Autodesk Inventor part; units mm, degrees
ref_plane "YZ Plane" through (0, 0, 0) normal (1, 0, 0) x (0, 1, 0)
ref_plane "XZ Plane" through (0, 0, 0) normal (0, 1, 0) x (-1, 0, 0)
ref_plane "XY Plane" through (0, 0, 0) normal (0, 0, 1) x (1, 0, 0)
sketch "スケッチ1" plane through (0, 0, 0) normal (0, 0, 1) x (1, 0, 0)
  line L0 (-21.75, 5.5) -> (-21.75, -5.5)
  line L1 (-21.75, -5.5) -> (-19.75, -5.5)
  line L2 (-21.75, 5.5) -> (-19.75, 5.5)
  line L3 (-19.75, 7.6) -> (-19.75, 10.5)
  line L4 (-19.75, 10.5) -> (19.75, 10.5)
  line L5 (19.75, 10.5) -> (19.75, 7.6)
  line L6 (-19.75, -7.6) -> (-19.75, -10.5)
  line L7 (-19.75, -10.5) -> (19.75, -10.5)
  line L8 (19.75, -10.5) -> (19.75, -7.6)
  line L9 (19.75, 5.5) -> (21.75, 5.5)
  line L10 (21.75, 5.5) -> (21.75, -5.5)
  line L11 (21.75, -5.5) -> (19.75, -5.5)
  line L12 (0, 0) -> (0, 10.5) construction
  line L13 (0, 0) -> (-21.75, 0) construction
  arc A0 (-19.75, 5.5) -> (-19.75, 7.6) centre (-19.75, 6.55) ccw
  arc A1 (-19.75, -7.6) -> (-19.75, -5.5) centre (-19.75, -6.55) ccw
  arc A2 (19.75, 7.6) -> (19.75, 5.5) centre (19.75, 6.55) ccw
  arc A3 (19.75, -5.5) -> (19.75, -7.6) centre (19.75, -6.55) ccw
  circle A4 centre (0, 0) radius 2.25
  dimension "d0" = 39.5
  dimension "d1" = 2
  dimension "d2" = 11
  dimension "d8" = 1.05
  dimension "d10" = 5
  dimension "d12" = 4.5
extrude "押し出し1" add sketch "スケッチ1" along normal blind 3
sketch "スケッチ2" plane through (0, 0, 0) normal (0, 0, -1) x (-1, 0, 0)
  circle A0 centre (0, 0) radius 2.25
  line L0 (-19.75, 10.5) -> (19.75, 10.5)
  line L1 (-21.75, -5.5) -> (-21.75, 5.5)
  arc A1 (6.3246, 3) -> (-6.3246, 3) centre (0, 0) ccw
  line L2 (-6.3246, 3) -> (-11.75, 3)
  line L3 (-11.75, 3) -> (-23.9536, 14.4408)
  line L4 (-23.9536, 14.4408) -> (23.9536, 14.4408)
  line L5 (23.9536, 14.4408) -> (11.75, 3)
  line L6 (11.75, 3) -> (6.3246, 3)
  line L7 (-19.75, 10.5) -> (19.75, 10.5) construction
  line L8 (0, 10.5) -> (0, 0) construction
  line L9 (0, 0) -> (-21.75, 0) construction
  arc A2 (-6.3246, -3) -> (6.3246, -3) centre (0, 0) ccw
  line L10 (-6.3246, -3) -> (-11.75, -3)
  line L11 (-11.75, -3) -> (-23.9536, -14.4408)
  line L12 (-23.9536, -14.4408) -> (23.9536, -14.4408)
  line L13 (23.9536, -14.4408) -> (11.75, -3)
  line L14 (11.75, -3) -> (6.3246, -3)
  dimension "d17" = 7
  dimension "d19" = 3
  dimension "d38" = 8
extrude "押し出し2" cut sketch "スケッチ2" against normal blind 10 contours L3 L4 L5 L0 | L0 L5 L6 A1 L2 L3 | A2 L14 L13 L12 L11 L10
fillet "フィレット1" radius 2 8 edges at (6.3246, 3, 1.5) (-6.3246, 3, 1.5) (6.3246, -3, 1.5) (-6.3246, -3, 1.5) (11.75, -3, 1.5) (11.75, 3, 1.5) (-11.75, 3, 1.5) (-11.75, -3, 1.5)
sketch "スケッチ3" plane through (0, 0, 3) normal (0, 0, 1) x (1, 0, 0)
  circle A0 centre (0, 0) radius 2.25
  line L0 (2.75, 1.5877) -> (2.75, -1.5877)
  line L1 (2.75, -1.5877) -> (0, -3.1754)
  line L2 (0, -3.1754) -> (-2.75, -1.5877)
  line L3 (-2.75, -1.5877) -> (-2.75, 1.5877)
  line L4 (-2.75, 1.5877) -> (0, 3.1754)
  line L5 (0, 3.1754) -> (2.75, 1.5877)
  line L6 (0, 3.187) -> (-2.76, 1.5935)
  line L7 (-2.76, 1.5935) -> (-2.76, -1.5935)
  line L8 (-2.76, -1.5935) -> (0, -3.187)
  line L9 (0, -3.187) -> (2.76, -1.5935)
  line L10 (2.76, -1.5935) -> (2.76, 1.5935)
  line L11 (2.76, 1.5935) -> (0, 3.187)
  circle A1 centre (0, 2.137) radius 1.05
  circle A2 centre (-1.8507, 1.0685) radius 1.05
  circle A3 centre (-1.8507, -1.0685) radius 1.05
  circle A4 centre (0, -2.137) radius 1.05
  circle A5 centre (1.8507, -1.0685) radius 1.05
  circle A6 centre (1.8507, 1.0685) radius 1.05
  point P0 (-2.76, 1.5935)
  point P1 (-2.76, -1.5935)
  point P2 (0, -3.187)
  point P3 (2.76, -1.5935)
  point P4 (2.76, 1.5935)
  dimension "d47" = 2.1
  dimension "d46" = 5.5
  dimension "d48" = 0.01
  dimension "d51" = 360
extrude "押し出し3" cut sketch "スケッチ3" against normal blind 2.2
equation "\"d2\" = d3"
equation "\"d10\" = d27"
properties part number "足首_サブフレーム_1_3" material "アルミニウム 2014-T4"
Here's how the part is built. I have some questions about the finished solid (model axes, mm). A direction names the side the tool comes from. Coordinates: 2 decimals unless noted, no trailing zeros. Write each loop counter-clockwise with the first axis right and the second up, starting at its lowest first coordinate (ties: lowest second). Pieces come first, ordered by that corner, then holes.
Item 1: I want a section at D-D on y = 8. Write out the boundary of the cut face in (x, z).
Item 2: If I drill on line 1 (X direction, y = 0, z = 0.25); line 2 (X direction, y = 1, z = 2.65); line 3 (Y direction, x = -9.5, z = 0.85), over which ranges is the centre line in solid material (lowest first)?
Item 3: On a 3-axis mill with a long thin cutter (end or side, diameter ignored), from which of +Z, -Z, +X, -X, +Y, -Y can I reach the whole of each face in a straight line? I mean faces 1 (the cylindrical face through (-6.53, -3.24, 1.52)), 2 (the flat face through (-16.09, 7.07, 1.48)), 3 (the flat face through (21, 5.5, 1)), 4 (the flat face through (-21, 5.5, 1)), 5 (the flat face through (-21, -5.5, 1)). Say none if no direction works.
Item 4: Will these pins go through, and if not, where does the flat tip stop? pin 1 (0.9 mm diameter, centred on x = -8.5, z = 1.5, fed in from -Y); pin 2 (12 mm diameter, centred on x = 16.5, y = -1, fed in from -Z); pin 3 (1.4 mm diameter, centred on y = -8.5, z = 2, fed in from +X); pin 4 (1 mm diameter, centred on x = 21, z = 1, fed in from +Y).
Item 5: I want a section at B-B on y = -9. Write out the boundary of the cut face in (x, z).
Item 6: If we mould it in two halves opening along Y, with no side actions, what happens to faces 6 (the flat face through (-1.387, -2.386, 1.915)), 7 (the cylindrical face through (-6.55, 3.23, 1.52)), 8 (the cylindrical face through (-2.768, -1.58, 1.915)), 9 (the cylindrical face through (-11.685, -3.136, 1.521))? For each: +Y half, -Y half, draft (parallel to the pull), parting line (faces both ways), or undercut.
Item 7: I want a section at C-C on x = -15.5. Write out the boundary of the cut face in (y, z).
Item 8: I want a section at A-A on y = -6.55. Write out the boundary of the cut face in (x, z).
Findings below:
1. outline: (-19.75, 0) - (-17.08, 0) - (-17.08, 3) - (-19.75, 3) - close; (17.08, 0) - (19.75, 0) - (19.75, 3) - (17.08, 3) - close
2. line 1: x = -21.75 to -2.25, 2.25 to 21.75
2. line 2: x = -21.75 to -2.9, 2.9 to 21.75
2. line 3: y = -3 to 3
3. face 1: +Z, -Z, -Y
3. face 2: +Z, -Z, +Y
3. face 3: +Z, -Z, +X, +Y
3. face 4: +Z, -Z, -X, +Y
3. face 5: +Z, -Z, -X, -Y
4. pin 1: stops at y = -3
4. pin 2: stops at z = 0
4. pin 3: stops at x = 19.75
4. pin 4: stops at y = 5.5
5. outline: (-19.75, 0) - (-18.15, 0) - (-18.15, 3) - (-19.75, 3) - close; (18.15, 0) - (19.75, 0) - (19.75, 3) - (18.15, 3) - close
6. face 6: undercut
6. face 7: +Y half
6. face 8: undercut
6. face 9: -Y half
7. outline: (-6.52, 0) - (6.52, 0) - (6.52, 3) - (-6.52, 3) - close
8. outline: (-18.7, 0) - (-15.54, 0) - (-15.54, 3) - (-18.7, 3) - close; (-2.47, 0) - (2.47, 0) - (2.47, 3) - (-2.47, 3) - close; (15.54, 0) - (18.7, 0) - (18.7, 3) - (15.54, 3) - close
